```python
from build123d import *

# Parameters (mm, degrees)
F0_W     = 120
F0_H     = 80
F0_R     = 5
F1_DEPTH = 10
F2_W     = 120
F2_H     = 10
F3_DEPTH = 55
F4_R     = 5
F5_DEPTH = 25
F7_DEPTH = 5
F9_DEPTH = 5


with BuildPart() as f1:
    # F0 (on Front) → F1 (new body)
    with BuildSketch(Plane.XZ):
        Rectangle(F0_W, F0_H)
        with Locations((-40, 20)):
            Circle(F0_R, mode=Mode.SUBTRACT)
        with Locations((40, 20)):
            Circle(F0_R, mode=Mode.SUBTRACT)
    extrude(amount=F1_DEPTH)

    # F2 (on Front) → F3 (join)
    with BuildSketch(Plane.XZ):
        with Locations((-0.077325, -19.974228)):
            Rectangle(F2_W, F2_H)
    extrude(amount=F3_DEPTH)

    # F4 (on face) → F5 (cut)
    with BuildSketch(Plane.XY.offset(-14.974228)):
        with Locations((-40.077325, -35)):
            Circle(F4_R)
        with Locations((39.922675, -35)):
            Circle(F4_R)
    extrude(amount=-F5_DEPTH, mode=Mode.SUBTRACT)

    # F6 (on Right) → F7 (join)
    with BuildSketch(Plane.YZ):
        Polygon((-10.15516, -15.042505), (-9.974833, 39.9572), (-55.15516, -15.042505), align=None)
    extrude(amount=-F7_DEPTH)

    # F8 (on Right) → F9 (join)
    with BuildSketch(Plane.YZ):
        Polygon((-10.064434, -14.750807), (-10.064434, 40.249193), (-55.064434, -14.750807), align=None)
    extrude(amount=F9_DEPTH)


solid = f1.part
```
Model file for the job. Use its own axes, mm. A direction names the side the tool comes from. Round coordinates to 2 decimals unless told otherwise and drop trailing zeros. Write each loop counter-clockwise with the first axis right and the second up, starting at its lowest first coordinate (ties: lowest second). Pieces come first, ordered by that corner, then holes. Notation, with made-up numbers: M -23.75,-6.75 L -11.75,-6.75 A18 ccw -11.75,23.25 Z; hole C -33,4 d7. An arc over 180 degrees is marked long. Put each result on its own line as item: value.
Item 1: Probe L1, parallel to Z at x = -40, y = -4.25; L2, parallel to X at y = -32, z = -24; L3, parallel to Y at x = -27, z = -18. List the from-to ranges inside material, lowest first. Write a range as from..to.
Responses:
L1: -40..15, 25..40
L2: -60.08..-44.08, -36.08..35.92, 43.92..59.92
L3: -55..0
Item 2: Cut at D-D (z = -18). List the corners of the cut face in (x, y).
Responses:
outline: M -60.08,-55 L 59.92,-55 L 59.92,-10 L 60,-10 L 60,0 L -60.08,0 Z; hole C -40.08,-35 d10; hole C 39.92,-35 d10
Item 3: Cut at B-B (y = -37). List the corners of the cut face in (x, z), and give its area (3 significant figures).
Responses:
outline: M -60.08,-24.97 L -44.66,-24.97 L -44.66,-14.97 L -60.08,-14.97 Z; M -35.49,-24.97 L 35.34,-24.97 L 35.34,-14.97 L 0,-14.97 L 0,-14.75 L 5,-14.75 L 5,7.33 L 0,7.33 L 0,7.06 L -5,7.06 L -5,-14.97 L -35.49,-14.97 Z; M 44.51,-24.97 L 59.92,-24.97 L 59.92,-14.97 L 44.51,-14.97 Z
area: 1,240 mm²
Item 4: Flat gauge pins, fed straight in: P1, Ø11, axis at y = -5.5, z = 16, coming from the -X side; P2, Ø3, axis at x = 0, y = -4.5, coming from the +Z side; P3, Ø13.5, axis at y = -42.5, z = 10, coming from the -X side. Where does each tip first touch, or does it go through?
Responses:
P1: x = -60
P2: z = 40
P3: x = -5
Item 5: Cut at C-C (x = -10). List the corners of the cut face in (y, z).
Responses:
outline: M -55,-24.97 L -10,-24.97 L -10,-40 L 0,-40 L 0,40 L -10,40 L -10,-14.97 L -55,-14.97 Z
Item 6: Mould opens along Y. For faces 1 (the cylindrical face through (34.928, -34.78, -19.904)), 2 (the flat face through (2.465, -32.249, 13.134)), 3 (the flat face through (5, -23, 1)) say: +Y half, -Y half, draft (parallel to the pull), parting line (faces both ways), or undercut.
Responses:
face 1: undercut
face 2: -Y half
face 3: draft
Item 7: Tool access for faces 4 (the flat face through (2, -33, -14.751)), 5 (the flat face through (-1, 0, 1)), 6 (the flat face through (-2.46, -32.26, 12.83)): list every direction of +Z, -Z, +X, -X, +Y, -Y with a clear straight run to the whole face (end or side of a thin tool).
Responses:
face 4: +X, -Y
face 5: +Z, -Z, +X, -X, +Y
face 6: +Z, -X, -Y
